from build123d import *

# Parameters (mm, degrees)
EXTRUDE_1_DEPTH     = 30
SKETCH_2_R          = 1.3
CUT_EXTRUDE_1_DEPTH = 30
SKETCH_3_W          = 5
SKETCH_3_H          = 10
EXTRUDE_2_DEPTH     = 2
EXTRUDE_3_DEPTH     = 2


with BuildPart() as part:
    # 草图1 → 凸台-拉伸1 (new body)
    with BuildSketch(Plane.XY):
        with BuildLine():
            Line((0, 3.5), (-2.1, 3.5))
            Line((-2.1, 3.5), (-8.1, 3.5))
            Line((-8.1, 3.5), (-8.1, 1.3))
            Line((-8.1, 1.3), (-2.1, 1.3))
            Line((-2.1, 1.3), (-2.1, -1.3))
            Line((-2.1, -1.3), (-8.1, -1.3))
            Line((-8.1, -1.3), (-8.1, -3.5))
            Line((-8.1, -3.5), (-2.1, -3.5))
            Line((-2.1, -3.5), (0, -3.5))
            Line((0, -3.5), (0, -5))
            Line((0, -5), (1.2510004, -5))
            ThreePointArc((1.2510004, -5), (2.5, -2.4), (3.7489996, -5))
            Line((3.7489996, -5), (5, -5))
            Line((5, -5), (5, -1.2489996))
            ThreePointArc((5, -1.2489996), (2.4, 0), (5, 1.2489996))
            Line((5, 1.2489996), (5, 5))
            Line((5, 5), (3.7489996, 5))
            ThreePointArc((3.7489996, 5), (2.5, 2.4), (1.2510004, 5))
            Line((1.2510004, 5), (0, 5))
            Line((0, 5), (0, 3.5))
        make_face()
    extrude(amount=EXTRUDE_1_DEPTH)

    # 草图2 → 切除-拉伸1 (cut)
    with BuildSketch(Plane.XZ.offset(3.5)):
        with Locations((-5.099947381, 15.002748372)):
            Circle(SKETCH_2_R)
        with Locations((-5.099947381, 7.501374186)):
            Circle(SKETCH_2_R)
        with Locations((-5.099947381, 22.502748372)):
            Circle(SKETCH_2_R)
    extrude(amount=-CUT_EXTRUDE_1_DEPTH, mode=Mode.SUBTRACT)

    # 草图3 → 凸台-拉伸2 (add)
    with BuildSketch(Plane.XY.offset(30)):
        with Locations((2.5, 0)):
            Rectangle(SKETCH_3_W, SKETCH_3_H)
    extrude(amount=-EXTRUDE_2_DEPTH)

    # 草图4 → 凸台-拉伸3 (add)
    with BuildSketch(Plane(origin=(0, 0, 0), x_dir=(-1, 0, 0), z_dir=(0, 0, -1))):
        with BuildLine():
            Line((0, 3.5), (0, 5))
            Line((0, 5), (-1.2510004, 5))
            ThreePointArc((-1.2510004, 5), (-2.5, 2.4), (-3.7489996, 5))
            Line((-3.7489996, 5), (-5, 5))
            Line((-5, 5), (-5, 1.2489996))
            ThreePointArc((-5, 1.2489996), (-2.4, 0), (-5, -1.2489996))
            Line((-5, -1.2489996), (-5, -5))
            Line((-5, -5), (-3.7489996, -5))
            ThreePointArc((-3.7489996, -5), (-2.5, -2.4), (-1.2510004, -5))
            Line((-1.2510004, -5), (0, -5))
            Line((0, -5), (0, -3.5))
            Line((0, -3.5), (0, 3.5))
        make_face()
        with BuildLine():
            Line((-1.2510004, 5), (-3.7489996, 5))
            ThreePointArc((-3.7489996, 5), (-2.5, 2.4), (-1.2510004, 5))
        make_face()
        with BuildLine():
            ThreePointArc((-5, -1.2489996), (-2.4, 0), (-5, 1.2489996))
            Line((-5, 1.2489996), (-5, -1.2489996))
        make_face()
        with BuildLine():
            Line((-3.7489996, -5), (-1.2510004, -5))
            ThreePointArc((-1.2510004, -5), (-2.5, -2.4), (-3.7489996, -5))
        make_face()
    extrude(amount=-EXTRUDE_3_DEPTH)


solid = part.part
Verification items for the finished model (mm, model axes). A direction names the side the tool comes from. Coordinates: 2 decimals unless noted, no trailing zeros. Order: outer loops, then holes, each group sorted by start corner. A loop starts at its lowest first (then second) coordinate and runs counter-clockwise, first axis right, second up. Notation, with made-up numbers: M 64,0 L 78,0 A21 cw 78,30 Z; hole C 17.25,18 d2. An arc over 180 degrees is marked long. One line per item, written item: value. Start each with the question number.
Item 1: Mould release check, pull along X, two halves, no side actions. Record for faces 4 (the cylindrical face through (2.45, -2.4, 14.82)), 5 (the flat face through (-2.1, 0, 15)), 6 (the flat face through (0, 0, 30)): released by +X, released by -X, zero draft, split by the parting line, or undercut.
Item 2: Gauge pin test, flat ends, axial feed: pin 1 (0.8 mm diameter, centred on y = -0.5, z = 15.5, fed in from -X); pin 2 (3 mm diameter, centred on x = -5, z = 24, fed in from -Y); pin 3 (3 mm diameter, centred on x = -5.1, z = 22.5, fed in from +Y). Record the tip position at first contact, or that the pin passes through.
Item 3: Sectioned sample at D-D (y = -2). Enter the section's corners in (x, z).
Item 4: Sectioned sample at A-A (y = 4). Enter the section's corners in (x, z), then the cut area to 3 significant figures.
Item 5: Sectioned sample at B-B (x = -3.25). Enter the section's corners in (y, z).
Item 6: Scan lines: probe 1 along Y at (x, z) = (-5.75, 11.75); probe 2 along Z at (x, y) = (-4, 2.75); probe 3 along X at (y, z) = (-4, 21). Record each from-to range of solid material in increasing order.
Item 7: Sectioned sample at C-C (z = 14). Enter the section's corners in (x, y).
Item 8: Access from +Z, -Z, +X, -X, +Y, -Y to the whole of each face (thin tool, end or side, straight path). Record for faces 1 (the flat face through (1, -5, 15)), 2 (the flat face through (2, -4, 28)), 3 (the flat face through (-3, -3.5, 15)).
Conclusion:
1. face 4: undercut
1. face 5: released by -X
1. face 6: zero draft
2. pin 1: stops at x = -2.1
2. pin 2: stops at y = -3.5
2. pin 3: stops at y = 3.5
3. outline: M -8.1,0 L 5,0 L 5,30 L -8.1,30 Z; hole C -5.1,7.5 d2.6; hole C -5.1,15 d2.6; hole C -5.1,22.5 d2.6
4. outline: M 0,0 L 5,0 L 5,30 L 0,30 Z; hole M 0.9,2 L 4.1,2 L 4.1,28 L 0.9,28 Z
4. area: 66.8 mm^2
5. outline: M -3.5,0 L -1.3,0 L -1.3,30 L -3.5,30 Z; M 1.3,0 L 3.5,0 L 3.5,30 L 1.3,30 Z
6. probe 1: y = -3.5 to -1.3, 1.3 to 3.5
6. probe 2: z = 0 to 6.81, 8.19 to 14.31, 15.7 to 21.81, 23.2 to 30
6. probe 3: x = 0 to 0.9, 4.1 to 5
7. outline: M -8.1,-3.5 L -5.93,-3.5 L -5.93,-1.3 L -8.1,-1.3 Z; M -8.1,1.3 L -5.93,1.3 L -5.93,3.5 L -8.1,3.5 Z; M -4.27,-3.5 L 0,-3.5 L 0,-5 L 1.25,-5 A1.6 cw long 3.75,-5 L 5,-5 L 5,-1.25 A1.6 cw long 5,1.25 L 5,5 L 3.75,5 A1.6 cw long 1.25,5 L 0,5 L 0,3.5 L -4.27,3.5 L -4.27,1.3 L -2.1,1.3 L -2.1,-1.3 L -4.27,-1.3 Z
8. face 1: +Z, -Z, +X, -X, -Y
8. face 2: none
8. face 3: +Z, -Z, -X, -Y
